Model file for the job. Use its own axes, mm. Face numbers are marked on the shaded views. A direction names the side the tool comes from. Give positions to 0.01 mm unless a question says otherwise; leave off trailing zeros. Order: outer loops, then holes, each group sorted by start corner. A loop starts at its lowest first (then second) coordinate and runs counter-clockwise, first axis right, second up. Notation, with made-up numbers: (9.5, -3.5) - (60.5, -3.5) arc R13 cw to (60.5, 4.5) - close; hole circle Ø8 at (34.25, 55.25). An arc over 180 degrees is marked (long way). Return JSON: item names as keys, results as strings. Group by question number.
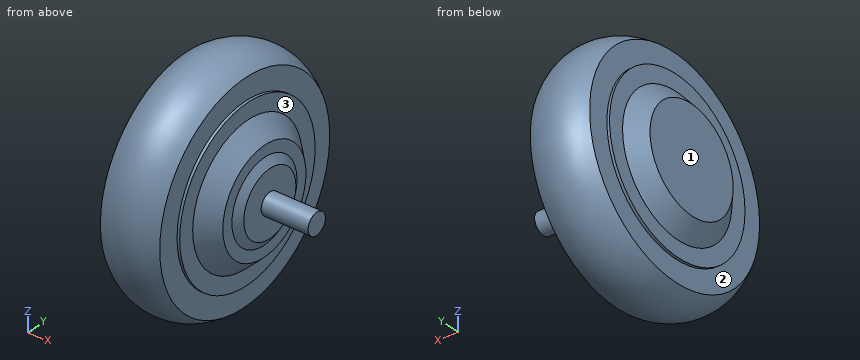
from build123d import *


with BuildPart() as part:
    # Croquis1 → Revolución1 (revolve)
    with BuildSketch(Plane.XY, mode=Mode.PRIVATE) as revoluci_n1_sk:
        with BuildLine():
            Line((-22, 165.221315178), (-22, 149.221315178))
            Line((-22, 149.221315178), (-24, 149.221315178))
            Line((-24, 149.221315178), (-24, 137.221315178))
            Line((-24, 137.221315178), (-34.6, 125))
            Line((-34.6, 125), (-34.6, 86.5))
            Line((-34.6, 86.5), (75.4, 86.5))
            Line((75.4, 86.5), (75.4, 94.5))
            Line((75.4, 94.5), (40.6, 94.5))
            Line((40.6, 94.5), (40.6, 110.6))
            Line((40.6, 110.6), (36.6, 116.6))
            Line((36.6, 116.6), (36.6, 125))
            Line((36.6, 125), (24, 137.221315178))
            Line((24, 137.221315178), (24, 149.221315178))
            Line((24, 149.221315178), (22, 149.221315178))
            Line((22, 149.221315178), (22, 165.221315178))
            ThreePointArc((22, 165.221315178), (0, 173), (-22, 165.221315178))
        make_face()
    revolve(revoluci_n1_sk.sketch.rotate(Axis((-34.6, 86.5, 0), (1, 0, 0)), 180), axis=Axis((-34.6, 86.5, 0), (1, 0, 0)))


solid = part.part
(1) Slice it at A-A (z = 0). Give the cut face in (x, y), and give its area (3 significant figures).
(2) Slice it at B-B (y = 86.5). Give the cut face in (x, z), and give its area (3 significant figures).
(3) Slice it at D-D (x = -12). Give the cut face in (y, z), and give its area (3 significant figures).
(4) Slice it at C-C (x = 4.5). Give the cut face in (y, z).
(5) Drop flat-ended pins along their axis: pin 1 Ø5 at (x, y) = (-7.5, 152.5) entering from +Z; pin 2 Ø8 at (x, y) = (23.5, 99) entering from -Z; pin 3 Ø4 at (x, y) = (27, 84) entering from +Z; pin 4 Ø1 at (x, y) = (38.5, 47) entering from -Z. Give the stop position or say it passes through.
(6) 3-axis set-ups, long thin cutter, end or side, ignore diameter. For the marked faces 1, 2 and 3: which of +Z, -Z, +X, -X, +Y, -Y reach the whole face in a straight line?
(7) Drill centre lines: L1, parallel to X at y = 115.5, z = 62.5; L2, parallel to X at y = 51.5, z = 50.5; L3, parallel to Y at x = 17, z = 4. Where is each one in solid material? Low to high.
Result set:
{
 "1": {"outline": "(-34.6, 48) - (-24, 35.78) - (-24, 23.78) - (-22, 23.78) - (-22, 7.78) arc R35 ccw to (22, 7.78) - (22, 23.78) - (24, 23.78) - (24, 35.78) - (36.6, 48) - (36.6, 56.4) - (40.6, 62.4) - (40.6, 78.5) - (75.4, 78.5) - (75.4, 94.5) - (40.6, 94.5) - (40.6, 110.6) - (36.6, 116.6) - (36.6, 125) - (24, 137.22) - (24, 149.22) - (22, 149.22) - (22, 165.22) arc R35 ccw to (-22, 165.22) - (-22, 149.22) - (-24, 149.22) - (-24, 137.22) - (-34.6, 125) - close", "area": "10,700 mm²"},
 "2": {"outline": "(-34.6, -38.5) - (-24, -50.72) - (-24, -62.72) - (-22, -62.72) - (-22, -78.72) arc R35 ccw to (22, -78.72) - (22, -62.72) - (24, -62.72) - (24, -50.72) - (36.6, -38.5) - (36.6, -30.1) - (40.6, -24.1) - (40.6, -8) - (75.4, -8) - (75.4, 8) - (40.6, 8) - (40.6, 24.1) - (36.6, 30.1) - (36.6, 38.5) - (24, 50.72) - (24, 62.72) - (22, 62.72) - (22, 78.72) arc R35 ccw to (-22, 78.72) - (-22, 62.72) - (-24, 62.72) - (-24, 50.72) - (-34.6, 38.5) - close", "area": "10,700 mm²"},
 "3": {"outline": "circle Ø168.76 at (86.5, 0)", "area": "22,400 mm²"},
 "4": {"outline": "circle Ø172.42 at (86.5, 0)"},
 "5": {"pin 1": "stops at z = 57.64", "pin 2": "stops at z = -79.66", "pin 3": "stops at z = 49.69", "pin 4": "passes through"},
 "6": {"face 1": "+Z, -Z, -X, +Y, -Y", "face 2": "-X", "face 3": "+X"},
 "7": {"L1": "x = -22 to 22", "L2": "x = -24 to 24", "L3": "y = 4.5 to 168.5"}
}
